Source: CAD feature listing. Evaluate the final solid. Frame: model axes, mm. A direction names the side the tool comes from. Give positions to 0.01 mm unless a question says otherwise; leave off trailing zeros. Order: outer loops, then holes, each group sorted by start corner. A loop starts at its lowest first (then second) coordinate and runs counter-clockwise, first axis right, second up. Notation, with made-up numbers: M 77,-23.75 L 86,-23.75 A19 cw 86,-7.75 Z; hole C 30,-34.75 d5. An arc over 180 degrees is marked long. Return JSON: item names as keys, results as strings.
from build123d import *

# Parameters (mm, degrees)
SKETCH1_W           = 35
SKETCH1_H           = 80
BOSS_EXTRUDE1_DEPTH = 7
SKETCH2_W           = 6
SKETCH2_H           = 4.5
SKETCH2_R           = 1
BOSS_EXTRUDE2_DEPTH = 16.55
SKETCH3_R           = 5
CUT_EXTRUDE1_DEPTH  = 7
CUT_EXTRUDE2_DEPTH  = 15
SKETCH5_W           = 8
SKETCH5_H           = 80
SKETCH5_R           = 2
BOSS_EXTRUDE3_DEPTH = 7


with BuildPart() as part:
    # Sketch1 → Boss-Extrude1 (new body)
    with BuildSketch(Plane.XY):
        Rectangle(SKETCH1_W, SKETCH1_H)
    extrude(amount=BOSS_EXTRUDE1_DEPTH)

    # Sketch2 → Boss-Extrude2 (add)
    with BuildSketch(Plane.XY.offset(7)):
        with Locations((0, 8.75)):
            Rectangle(SKETCH2_W, SKETCH2_H)
        with Locations((0, 8.75)):
            Circle(SKETCH2_R, mode=Mode.SUBTRACT)
        with Locations((0, -19.05)):
            Rectangle(SKETCH2_W, SKETCH2_H)
        with Locations((0, -19.05)):
            Circle(SKETCH2_R, mode=Mode.SUBTRACT)
    extrude(amount=BOSS_EXTRUDE2_DEPTH)

    # Sketch3 → Cut-Extrude1 (cut)
    with BuildSketch(Plane.XY.offset(7)):
        Circle(SKETCH3_R)
    extrude(amount=-CUT_EXTRUDE1_DEPTH, mode=Mode.SUBTRACT)

    # Sketch4 → Cut-Extrude2 (cut)
    with BuildSketch(Plane.XY.offset(7)):
        with BuildLine():
            Line((-11.12, 36), (-11.12, -35.5))
            ThreePointArc((-11.12, -35.5), (-13.12, -37.5), (-15.12, -35.5))
            Line((-15.12, -35.5), (-15.12, 36))
            ThreePointArc((-15.12, 36), (-13.12, 38), (-11.12, 36))
        make_face()
        with BuildLine():
            Line((11.12, 36), (11.12, -35.5))
            ThreePointArc((11.12, -35.5), (13.12, -37.5), (15.12, -35.5))
            Line((15.12, -35.5), (15.12, 36))
            ThreePointArc((15.12, 36), (13.12, 38), (11.12, 36))
        make_face()
    extrude(amount=-CUT_EXTRUDE2_DEPTH, mode=Mode.SUBTRACT)

    # Sketch5 → Boss-Extrude3 (add)
    with BuildSketch(Plane.XY.offset(7)):
        with Locations((21.5, 0)):
            Rectangle(SKETCH5_W, SKETCH5_H)
        with Locations((21.5, 35)):
            Circle(SKETCH5_R, mode=Mode.SUBTRACT)
        with Locations((21.5, 25)):
            Circle(SKETCH5_R, mode=Mode.SUBTRACT)
        with Locations((21.5, 15)):
            Circle(SKETCH5_R, mode=Mode.SUBTRACT)
        with Locations((21.5, 5)):
            Circle(SKETCH5_R, mode=Mode.SUBTRACT)
        with Locations((21.5, -5)):
            Circle(SKETCH5_R, mode=Mode.SUBTRACT)
        with Locations((21.5, -15)):
            Circle(SKETCH5_R, mode=Mode.SUBTRACT)
        with Locations((21.5, -25)):
            Circle(SKETCH5_R, mode=Mode.SUBTRACT)
        with Locations((21.5, -35)):
            Circle(SKETCH5_R, mode=Mode.SUBTRACT)
    boss_extrude3 = extrude(amount=-BOSS_EXTRUDE3_DEPTH)

    # Mirror1: Boss-Extrude3 across plane
    add(boss_extrude3.mirror(Plane(origin=(0, 0, 0), x_dir=(0, 0, 1), z_dir=(1, 0, 0))))


solid = part.part
1. Ray query, probe 1 along X at (y, z) = (8, 3); probe 2 along Y at (x, z) = (0, 16); probe 3 along Z at (x, y) = (11, 8). Return the intervals inside material, ascending.
Evaluation:
{"probe 1": "x = -25.5 to -15.12, -11.12 to 11.12, 15.12 to 25.5", "probe 2": "y = -21.3 to -20.05, -18.05 to -16.8, 6.5 to 7.75, 9.75 to 11", "probe 3": "z = 0 to 7"}
2. Section query A-A (y = 25). Return loops of the section in (x, z), then the cut area to 3 significant figures.
Evaluation:
{"outline": "M -25.5,0 L -23.5,0 L -23.5,7 L -25.5,7 Z; M -19.5,0 L -15.12,0 L -15.12,7 L -19.5,7 Z; M -11.12,0 L 11.12,0 L 11.12,7 L -11.12,7 Z; M 15.12,0 L 19.5,0 L 19.5,7 L 15.12,7 Z; M 23.5,0 L 25.5,0 L 25.5,7 L 23.5,7 Z", "area": "245 mm^2"}
3. Set-up query: faces 1 (the face through (-0.13, 9.74, 15.16)), 2 (the face through (-3, 9, 15)), 3 (the face through (0, 10, 23.55)), 4 (the face through (13.1, -37.5, 3.5)). Return all of +Z, -Z, +X, -X, +Y, -Y with unobstructed straight access to the full face (end or side cutting, diameter ignored); none if empty.
Evaluation:
{"face 1": "+Z", "face 2": "+Z, -X, +Y, -Y", "face 3": "+Z, +X, -X, +Y, -Y", "face 4": "+Z, -Z"}
4. Section query D-D (z = 14.25). Return loops of the section in (x, y).
Evaluation:
{"outline": "M -3,-21.3 L 3,-21.3 L 3,-16.8 L -3,-16.8 Z; M -3,6.5 L 3,6.5 L 3,11 L -3,11 Z; hole C 0,-19.05 d2; hole C 0,8.75 d2"}
5. Section query B-B (z = 6). State how many separate pieces and enclosed holes the cut face has, then the cut area to 3 significant figures.
Evaluation:
{"separate pieces": "1", "enclosed holes": "19", "area": "3,200 mm^2"}
6. First-contact query: pin 1 (6.5 mm diameter, centred on x = -1, z = 14, fed in from -Y); pin 2 (5 mm diameter, centred on y = 9, z = 18, fed in from +X); pin 3 (6 mm diameter, centred on x = 4.5, y = 29.5, fed in from +Z); pin 4 (4 mm diameter, centred on x = 5.5, z = 14.5, fed in from -Y). Flat tips, straight axial feed; report the tip coordinate or a pass-through.
Evaluation:
{"pin 1": "stops at y = -21.3", "pin 2": "stops at x = 3", "pin 3": "stops at z = 7", "pin 4": "passes through"}
7. Section query C-C (x = 13.12). Return loops of the section in (y, z), then the cut area to 3 significant figures.
Evaluation:
{"outline": "M -40,0 L -37.5,0 L -37.5,7 L -40,7 Z; M 38,0 L 40,0 L 40,7 L 38,7 Z", "area": "31.5 mm^2"}
8. Draft query along X for faces 5 (the face through (3, -19, 15)), 6 (the face through (0, 6.5, 15)), 7 (the face through (0.46, -19.94, 15.16)). Return one class per face: pulls with the +X half, pulls with the -X half, needs draft (parallel to the pull), parting line crosses it, or undercut.
Evaluation:
{"face 5": "pulls with the +X half", "face 6": "needs draft", "face 7": "undercut"}
